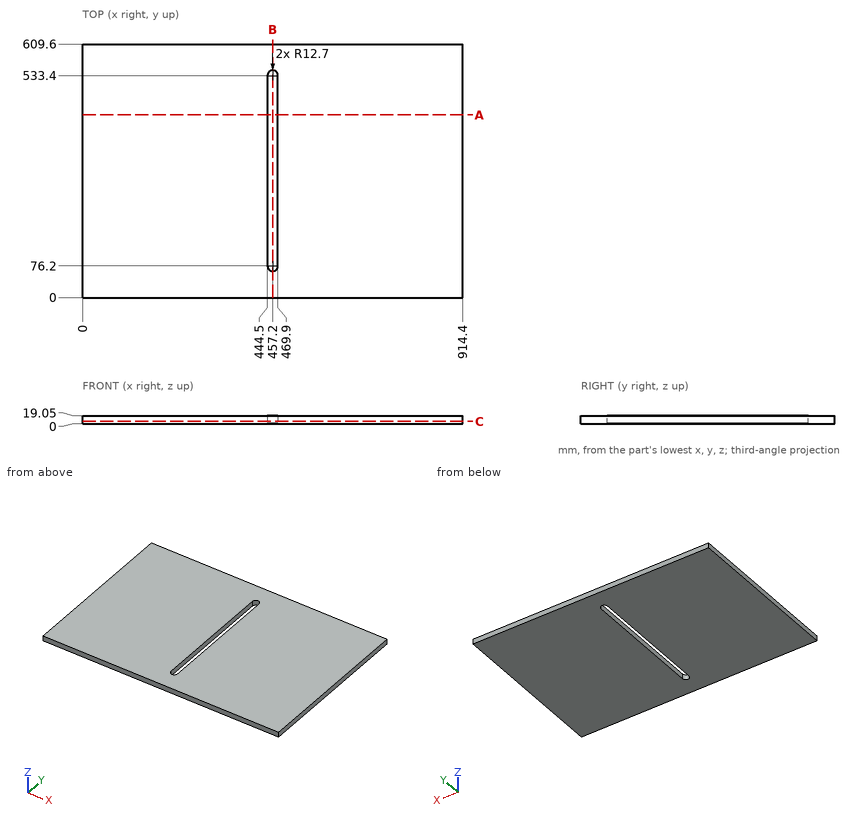
Check sheet for the drawn part. Datum: minimum x, y, z corner. Units: mm. Round coordinates to 2 decimals unless told otherwise and drop trailing zeros. Order: outer loops, then holes, each group sorted by start corner. A loop starts at its lowest first (then second) coordinate and runs counter-clockwise, first axis right, second up. Notation, with made-up numbers: (89, 4) -> (100, 4) arc R18 cw to (100, 36) -> close; hole circle Ø7 at (-11.5, -9). An arc over 180 degrees is marked (long way). Put each result on its own line as item: value. Start each with the question number.
(1) Section check C-C (z = 5). Enter the section's corners in (x, y), then the cut area to 3 significant figures.
(2) Material ranges on line 1 along X through (y, z) = (426.5, 7), recorded low to high.
(3) Section check B-B (x = 457.2). Enter the section's corners in (y, z).
(4) Section check A-A (y = 439.5). Enter the section's corners in (x, z), then the cut area to 3 significant figures.
Completed:
1. outline: (0, 0) -> (914.4, 0) -> (914.4, 609.6) -> (0, 609.6) -> close; hole (444.5, 76.2) arc R12.7 ccw to (469.9, 76.2) -> (469.9, 533.4) arc R12.7 ccw to (444.5, 533.4) -> close
1. area: 545,000 mm2
2. line 1: x = 0 to 444.5, 469.9 to 914.4
3. outline: (0, 0) -> (63.5, 0) -> (63.5, 19.05) -> (0, 19.05) -> close; (546.1, 0) -> (609.6, 0) -> (609.6, 19.05) -> (546.1, 19.05) -> close
4. outline: (0, 0) -> (444.5, 0) -> (444.5, 19.05) -> (0, 19.05) -> close; (469.9, 0) -> (914.4, 0) -> (914.4, 19.05) -> (469.9, 19.05) -> close
4. area: 16,900 mm2
